Build history of the part. All positions in model axes, mm. Face numbers are marked on the shaded views. A direction names the side the tool comes from. Coordinates: 2 decimals unless noted, no trailing zeros. Loops run counter-clockwise (first coordinate to the right, second up) from the corner with the lowest first, then second, coordinate; pieces in that order, holes last.
(1) Slice it at A-A (z = -35.4). Give the cut face in (x, y), and give its area (3 significant figures).
(2) Two-plate mould, pull along X, no slides. Class the marked faces 3, 4 and 5: pulls with the +X half, pulls with the -X half, needs draft (parallel to the pull), parting line crosses it, or undercut.
(3) Wall check: L1, parallel to Z at x = 22.85, y = 0.35; L2, parallel to X at y = 7.75, z = -57; L3, parallel to X at y = 4.75, z = -5. Give the ranges that are in metal, low to high.
(4) Flat gauge pins, fed straight in: P1, Ø1, axis at y = 3.5, z = -62.5, coming from the +X side; P2, Ø13.5, axis at x = -9.5, z = -60, coming from the +Y side. Where does each tip first touch, or does it go through?
(5) Slice it at C-C (x = 22.85). Give the cut face in (y, z).
(6) Slice it at D-D (z = -21). Give the cut face in (x, y), and give its area (3 significant figures).
(7) Slice it at B-B (y = 2.75). Give the number of separate pieces and of enclosed holes in the cut face, and give its area (3 significant figures).
(8) Tool access for the marked faces 1 and 2: list every direction of +Z, -Z, +X, -X, +Y, -Y with a clear straight run to the whole face (end or side of a thin tool).
from build123d import *

# Parameters (mm, degrees)
SKETCH1_W                    = 2.5
SKETCH1_H                    = 12
BOSS_EXTRUDE1_DEPTH          = 0.5
BOSS_EXTRUDE2_DEPTH          = 9.55
F_3_0_3_DIAMETER_HOLE1_D     = 3
F_3_0_3_DIAMETER_HOLE1_DEPTH = 12
F_3_0_3_DIAMETER_HOLE1_TIP   = 0.901290929


with BuildPart() as part:
    # Sketch1 → Boss-Extrude1 (new body)
    with BuildSketch(Plane(origin=(0, 0, 0), x_dir=(1, 0, 0), z_dir=(0, 1, 0))):
        Polygon((-21.75, 31.85), (0, 31.85), (0, 76.35), (-26.25, 76.35), (-26.25, 53.35), (-26.25, 41.35), (-26.25, 31.85), align=None)
        Polygon((0, 76.35), (0, 31.85), (21.75, 31.85), (26.25, 31.85), (26.25, 76.35), align=None)
        with Locations((-27.5, 47.35)):
            Rectangle(SKETCH1_W, SKETCH1_H)
    extrude(amount=BOSS_EXTRUDE1_DEPTH)

    # Sketch1_3 → Boss-Extrude2 (add)
    with BuildSketch(Plane(origin=(0, 0, 0), x_dir=(1, 0, 0), z_dir=(0, 1, 0))):
        with BuildLine():
            Line((-28.75, 73.35), (-28.75, 53.35))
            Line((-28.75, 53.35), (-26.25, 53.35))
            Line((-26.25, 53.35), (-26.25, 79.35))
            Line((-26.25, 79.35), (-30.25, 79.35))
            ThreePointArc((-30.25, 79.35), (-33.25, 76.35), (-30.25, 73.35))
            Line((-30.25, 73.35), (-28.75, 73.35))
        make_face()
        with BuildLine():
            Line((26.25, 79.35), (26.25, 31.85))
            Line((26.25, 31.85), (21.75, 31.85))
            Line((21.75, 31.85), (21.75, 0))
            Line((21.75, 0), (28.75, 0))
            Line((28.75, 0), (28.75, 73.35))
            Line((28.75, 73.35), (30.25, 73.35))
            ThreePointArc((30.25, 73.35), (33.25, 76.35), (30.25, 79.35))
            Line((30.25, 79.35), (26.25, 79.35))
        make_face()
        Polygon((-26.25, 31.85), (-26.25, 41.35), (-28.75, 41.35), (-28.75, 0), (-21.75, 0), (-21.75, 31.85), align=None)
    extrude(amount=BOSS_EXTRUDE2_DEPTH)

    # 3.0 _3_ Diameter Hole1
    with Locations(Plane(origin=(0, 0, 0), x_dir=(-1, 0, 0), z_dir=(0, -1, 0))):
        with Locations((-22.85, 73.45), (22.85, 73.45), (26, 29.35), (22.85, 35.4), (-22.85, 35.4), (-26, 29.35), (-26, 3), (26, 3), (-30.25, 76.35), (30.25, 76.35)):
            Hole(F_3_0_3_DIAMETER_HOLE1_D / 2, depth=F_3_0_3_DIAMETER_HOLE1_DEPTH)
            with Locations((0, 0, -(F_3_0_3_DIAMETER_HOLE1_DEPTH + F_3_0_3_DIAMETER_HOLE1_TIP / 2))):  # 118° drill point
                Cone(0, F_3_0_3_DIAMETER_HOLE1_D / 2, F_3_0_3_DIAMETER_HOLE1_TIP, mode=Mode.SUBTRACT)


solid = part.part
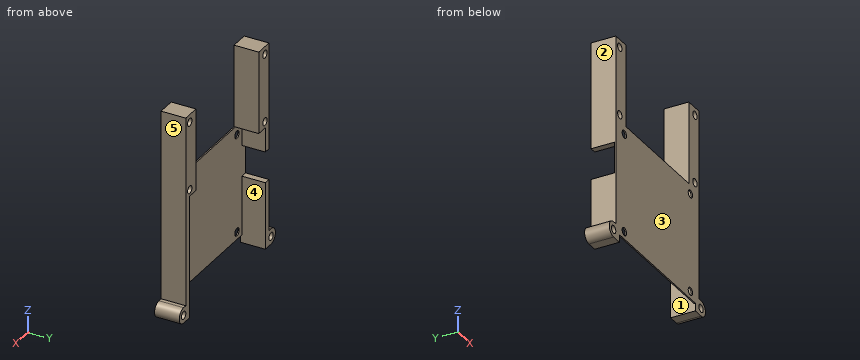
Response values:
1. outline: (-28.75, 0) - (-24.35, 0) - (-24.35, 0.5) - (-26.25, 0.5) - (-26.25, 9.55) - (-28.75, 9.55) - close; (-21.35, 0) - (21.35, 0) - (21.35, 0.5) - (-21.35, 0.5) - close; (24.35, 0) - (28.75, 0) - (28.75, 9.55) - (26.25, 9.55) - (26.25, 0.5) - (24.35, 0.5) - close
1. area: 71.0 mm2
2. face 3: needs draft
2. face 4: undercut
2. face 5: pulls with the +X half
3. L1: z = -76.35 to -74.95, -71.95 to -36.9, -33.9 to 0
3. L2: x = -28.75 to -26.25, 26.25 to 28.75
3. L3: x = -28.75 to -21.75, 21.75 to 28.75
4. P1: stops at x = 28.75
4. P2: stops at y = 0.5
5. outline: (0, -76.35) - (0.5, -76.35) - (0.5, -74.95) - (0, -74.95) - close; (0, -71.95) - (0.5, -71.95) - (0.5, -36.9) - (0, -36.9) - close; (0, -33.9) - (0.5, -33.9) - (0.5, -31.85) - (9.55, -31.85) - (9.55, 0) - (0, 0) - close
6. outline: (-28.75, 0) - (-21.75, 0) - (-21.75, 9.55) - (-28.75, 9.55) - close; (21.75, 0) - (28.75, 0) - (28.75, 9.55) - (21.75, 9.55) - close
6. area: 134 mm2
7. separate pieces: 3
7. enclosed holes: 6
7. area: 657 mm2
8. face 1: -Z, +Y
8. face 2: +Z, -X, +Y, -Y
